Here's how the part is built. I have some questions about the finished solid (model axes, mm). A direction names the side the tool comes from. Round coordinates to 2 decimals unless told otherwise and drop trailing zeros. Loops run counter-clockwise (first coordinate to the right, second up) from the corner with the lowest first, then second, coordinate; pieces in that order, holes last. Notation, with made-up numbers: M -36.75,-22 L 20.25,-22 A12 cw 20.25,-9 Z; hole C -9,11.5 d2. An arc over 180 degrees is marked long. Answer as a JSON object with one key per item and string values.
from build123d import *

# Parameters (mm, degrees)
F2_SIZE  = 0.5
F3_SIZE  = 0.5
F6_DEPTH = 2.9


with BuildPart() as f1:
    # F0 (on Front) → F1 (revolve)
    with BuildSketch(Plane.XZ):
        with BuildLine():
            add(Edge.make_bspline(
                [(1.5, 2.4199453937), (3.8369755758, 2.1967958582), (6.7693715651, 1.4854960684), (7.95, 0)],
                knots=[1.568331731, 1.568331731, 1.568331731, 1.568331731, 8.3338166527, 8.3338166527, 8.3338166527, 8.3338166527], degree=3))
            Line((7.95, 0), (10.65, 0))
            Line((10.65, 0), (10.65, 2.6))
            Line((10.65, 2.6), (6.05, 2.6))
            Line((6.05, 2.6), (6.05, 4))
            Line((6.05, 4), (3.9, 4))
            Line((3.9, 4), (3.9, 6.9))
            Line((3.9, 6.9), (0, 6.9))
            Line((0, 6.9), (0, 2.9199453937))
            Line((0, 2.9199453937), (1.5, 2.9199453937))
            Line((1.5, 2.9199453937), (1.5, 2.4199453937))
        make_face()
    revolve(axis=Axis((0, 0, 3.45), (0, 0, -1)))

    # F2
    f2_edges = [f1.edges().sort_by_distance(p)[0] for p in [
        (-3.9, 0, 6.9),
    ]]
    chamfer(f2_edges, length=F2_SIZE)

    # F3
    f3_edges = [f1.edges().sort_by_distance(p)[0] for p in [
        (-10.65, 0, 0),
    ]]
    chamfer(f3_edges, length=F3_SIZE)

    # F5 (on offset) → F6 (cut)
    with BuildSketch(Plane.XY.offset(6.9)):
        with BuildLine():
            ThreePointArc((0.3, -2.9849623113), (2.2248595461, -2.0124611797), (3, 0))
            ThreePointArc((3, 0), (2.2248595461, 2.0124611797), (0.3, 2.9849623113))
            Line((0.3, 2.9849623113), (0.3, 0))
            Line((0.3, 0), (0.3, -2.9849623113))
        make_face()
        with BuildLine():
            Line((0.3, 0), (0.3, 2.9849623113))
            ThreePointArc((0.3, 2.9849623113), (0, 3), (-0.3, 2.9849623113))
            Line((-0.3, 2.9849623113), (-0.3, 0))
            Line((-0.3, 0), (0, 0))
            Line((0, 0), (0.3, 0))
        make_face()
        with BuildLine():
            ThreePointArc((-0.3, 2.9849623113), (0, 3), (0.3, 2.9849623113))
            Line((0.3, 2.9849623113), (0.3, 4.0277631488))
            Line((0.3, 4.0277631488), (-0.3, 4.0277631488))
            Line((-0.3, 4.0277631488), (-0.3, 2.9849623113))
        make_face()
        with BuildLine():
            Line((0.3, -3.8517790381), (0.3, -2.9849623113))
            ThreePointArc((0.3, -2.9849623113), (0, -3), (-0.3, -2.9849623113))
            Line((-0.3, -2.9849623113), (-0.3, -3.8517790381))
            Line((-0.3, -3.8517790381), (0.3, -3.8517790381))
        make_face()
        with BuildLine():
            ThreePointArc((-0.3, -2.9849623113), (0, -3), (0.3, -2.9849623113))
            Line((0.3, -2.9849623113), (0.3, 0))
            Line((0.3, 0), (0, 0))
            Line((0, 0), (-0.3, 0))
            Line((-0.3, 0), (-0.3, -2.9849623113))
        make_face()
        with BuildLine():
            Line((-0.3, 0), (-0.3, 2.9849623113))
            ThreePointArc((-0.3, 2.9849623113), (-3, 0), (-0.3, -2.9849623113))
            Line((-0.3, -2.9849623113), (-0.3, 0))
        make_face()
    extrude(amount=-F6_DEPTH, mode=Mode.SUBTRACT)


solid = f1.part
Item 1: We'd pull the mould along X, two halves only. Please class faces 1 (the face through (5.589, 2.317, 3.31)), 2 (the face through (6.8, 4.5, 0)), 3 (the face through (-3, 0, 5)), 4 (the face through (-1.5, -0.07, 2.67)): +X half, -X half, draft (parallel to the pull), parting line (faces both ways), or undercut.
Solution:
{"face 1": "parting line", "face 2": "draft", "face 3": "undercut", "face 4": "undercut"}
Item 2: I want a section at A-A on z = 3.5. List the corners of the cut face in (x, y) for me.
Solution:
{"outline": "C 0,0 d12.1"}
Item 3: For faces 5 (the face through (3, 1, 6.9)), 6 (the face through (0.3, 3.4, 5.5)), 7 (the face through (2.583, -2.922, 5.217)), 8 (the face through (0, 0, 2.92)), which set-ups out of +Z, -Z, +X, -X, +Y, -Y let a thin tool reach every point of the face, with its end or its side?
Solution:
{"face 5": "+Z, +X, -X, +Y, -Y", "face 6": "+Z, +Y", "face 7": "+Z", "face 8": "-Z"}
Item 4: If I drill on L1, parallel to Y at x = 0, z = 2.65; L2, parallel to Z at x = 4.5, y = 9, over which ranges is the centre line in solid material (lowest first)? Write a range as from..to.
Solution:
{"L1": "y = -6.05..-1.5, 1.5..6.05", "L2": "z = 0..2.6"}
Item 5: For P1, Ø1, axis at y = -6, z = 1.5, coming from the +X side; P2, Ø2, axis at y = 2, z = 4, coming from the -X side; P3, Ø3, axis at x = -1, z = 5, coming from the +Y side, each with a flat end and sliding along its axis, tell me the tip position at first contact or that it passes through.
Solution:
{"P1": "stops at x = 9.12", "P2": "stops at x = -5.97", "P3": "stops at y = 6.05"}
